```python
from build123d import *

# Parameters (mm, degrees)
SKETCH1_W           = 55
SKETCH1_H           = 55
SKETCH1_W_2         = 12
SKETCH1_H_2         = 13.5
BOSS_EXTRUDE1_DEPTH = 8
SKETCH2_W           = 55
SKETCH2_H           = 55
BOSS_EXTRUDE7_DEPTH = 12
SKETCH2_5_W         = 23.6
SKETCH2_5_H         = 7
SKETCH2_5_W_2       = 47
BOSS_EXTRUDE8_DEPTH = 8
SKETCH6_R           = 3.15
CUT_EXTRUDE1_DEPTH  = 44.732139211
SKETCH7_W           = 24.995653022
SKETCH7_H           = 4
CUT_EXTRUDE3_DEPTH  = 4


with BuildPart() as part:
    # Sketch1 → Boss-Extrude1 (new body)
    with BuildSketch(Plane(origin=(0, 0, 0), x_dir=(1, 0, 0), z_dir=(0, 1, 0))):
        Rectangle(SKETCH1_W, SKETCH1_H)
        with Locations((0, 16.75)):
            Rectangle(SKETCH1_W_2, SKETCH1_H_2, mode=Mode.SUBTRACT)
        with Locations((17.5, 0)):
            Rectangle(SKETCH1_W_2, SKETCH1_H_2, mode=Mode.SUBTRACT)
        with Locations((-17.5, 0)):
            Rectangle(SKETCH1_W_2, SKETCH1_H_2, mode=Mode.SUBTRACT)
        with Locations((0, -16.75)):
            Rectangle(SKETCH1_W_2, SKETCH1_H_2, mode=Mode.SUBTRACT)
    extrude(amount=BOSS_EXTRUDE1_DEPTH)

    # Sketch2 → Boss-Extrude7 (add)
    with BuildSketch(Plane.XZ):
        Rectangle(SKETCH2_W, SKETCH2_H)
        Polygon((-23.5, 23.5), (-6, 23.5), (6, 23.5), (23.5, 23.5), (23.5, 6.75), (23.5, 3.5), (23.5, -3.5), (23.5, -6.75), (23.5, -23.5), (6, -23.5), (-6, -23.5), (-23.5, -23.5), (-23.5, -6.75), (-23.5, -3.5), (-23.5, 3.5), (-23.5, 6.75), align=None, mode=Mode.SUBTRACT)
    extrude(amount=BOSS_EXTRUDE7_DEPTH)

    # Sketch2_5 → Boss-Extrude8 (add)
    with BuildSketch(Plane.XZ):
        with Locations((-0.1, 16.75)):
            Rectangle(SKETCH2_5_W, SKETCH2_5_H)
        Rectangle(SKETCH2_5_W_2, SKETCH2_5_H)
        with Locations((-0.1, -16.75)):
            Rectangle(SKETCH2_5_W, SKETCH2_5_H)
    extrude(amount=BOSS_EXTRUDE8_DEPTH)

    # Sketch6 → Cut-Extrude1 (cut, through all)
    with BuildSketch(Plane.XZ.offset(12)):
        with Locations(Location((-23.5, 23.5, 0), (0, 0, 270))):
            Circle(SKETCH6_R)
        with Locations(Location((23.5, 23.5, 0), (0, 0, 270))):
            Circle(SKETCH6_R)
        with Locations(Location((-23.5, -23.5, 0), (0, 0, 270))):
            Circle(SKETCH6_R)
        with Locations(Location((23.5, -23.5, 0), (0, 0, 270))):
            Circle(SKETCH6_R)
    extrude(amount=-CUT_EXTRUDE1_DEPTH, mode=Mode.SUBTRACT)

    # Sketch7 → Cut-Extrude3 (cut)
    with BuildSketch(Plane(origin=(27.5, 0, 0), x_dir=(0, 0, -1), z_dir=(1, 0, 0))):
        with Locations((0, -10)):
            Rectangle(SKETCH7_W, SKETCH7_H)
    extrude(amount=-CUT_EXTRUDE3_DEPTH, mode=Mode.SUBTRACT)


solid = part.part
```
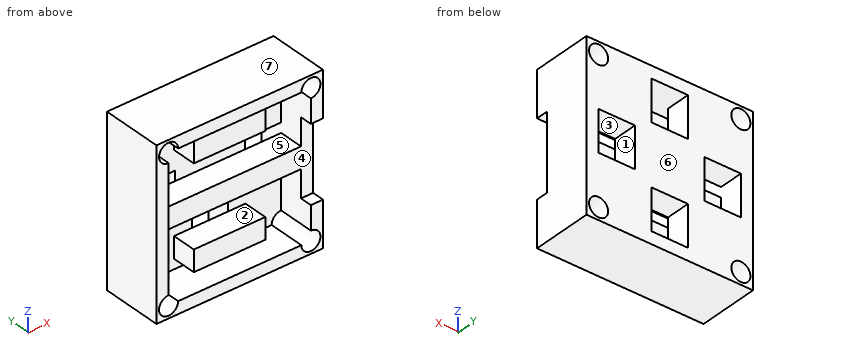
The listing builds one solid part. Answer for the finished solid, in the listing's coordinates (mm). Face numbers are marked on the shaded views. A direction names the side the tool comes from. Coordinates: 2 decimals unless noted, no trailing zeros. Order: outer loops, then holes, each group sorted by start corner. A loop starts at its lowest first (then second) coordinate and runs counter-clockwise, first axis right, second up. Notation, with made-up numbers: M 21.5,78.25 L 35.5,78.25 A33 ccw 35.5,117.25 Z; hole C 10.5,79 d8. An arc over 180 degrees is marked long. Answer as a JSON object with one key per item and string values. Group by question number.
1. Flat-ended cylindrical pins translate along their axes: P1, Ø5, axis at x = 18, z = 0, coming from the -Y side; P2, Ø5.5, axis at x = 0.5, z = -17, coming from the +Y side. Find the tip coordinate at first contact, or state that the pin passes through.
2. Determine the mould class of the marked faces 5, 6 and 7 for opening direction Z: released by +Z, released by -Z, zero draft, split by the parting line, or undercut.
3. A tool of negligible diameter and unlimited length cuts with its end or side. For the marked faces 1, 2, 3 and 4, from which of +Z, -Z, +X, -X, +Y, -Y can it reach the whole face along a straight path? Write none if from no direction.
4. Straight lines are drawn through the part: line 1 (Z direction, x = -8.5, y = -4.75); line 2 (X direction, y = 6.5, z = 3.5); line 3 (Z direction, x = 6, y = -10.25). For each, find the intervals that lie inside material, in ascending order.
5. Section A-A on x = 17 is taken. Write down the section's boundary in (y, z).
6. Section C-C on z = -6 is taken. Write down the section's boundary in (x, y).
7. Section D-D on x = -3.5 is taken. Write down the section's boundary in (y, z), then the cut area to 3 significant figures.
8. Section B-B on y = -2.25 is taken. Write down the section's boundary in (x, z).
Values follow:
{
 "1": {"P1": "y = -8", "P2": "y = 0"},
 "2": {"face 5": "undercut", "face 6": "zero draft", "face 7": "released by +Z"},
 "3": {"face 1": "+Y", "face 2": "-Y", "face 3": "+Y, -Y", "face 4": "+X, -Y"},
 "4": {"line 1": "-27.5 to -23.5, -20.25 to -13.25, -3.5 to 3.5, 13.25 to 20.25, 23.5 to 27.5", "line 2": "-27.5 to -23.5, -11.5 to 11.5, 23.5 to 27.5", "line 3": "-27.5 to -23.5, 23.5 to 27.5"},
 "5": {"outline": "M -12,-27.5 L 8,-27.5 L 8,-6.75 L 0,-6.75 L 0,-23.5 L -12,-23.5 Z; M -12,23.5 L 0,23.5 L 0,6.75 L 8,6.75 L 8,27.5 L -12,27.5 Z; M -8,-3.5 L 0,-3.5 L 0,3.5 L -8,3.5 Z"},
 "6": {"outline": "M -27.5,-12 L -23.5,-12 L -23.5,8 L -27.5,8 Z; M -11.5,0 L 11.5,0 L 11.5,8 L -11.5,8 Z; M 23.5,-8 L 27.5,-8 L 27.5,8 L 23.5,8 Z"},
 "7": {"outline": "M -12,-27.5 L 8,-27.5 L 8,-23.5 L -12,-23.5 Z; M -12,23.5 L 8,23.5 L 8,27.5 L -12,27.5 Z; M -8,-20.25 L 0,-20.25 L 0,-13.25 L -8,-13.25 Z; M -8,-3.5 L 0,-3.5 L 0,-10 L 8,-10 L 8,10 L 0,10 L 0,3.5 L -8,3.5 Z; M -8,13.25 L 0,13.25 L 0,20.25 L -8,20.25 Z", "area": "488 mm2"},
 "8": {"outline": "M -27.5,-27.5 L 27.5,-27.5 L 27.5,27.5 L -27.5,27.5 Z; M -11.9,-20.25 L 11.7,-20.25 L 11.7,-13.25 L -11.9,-13.25 Z; M -11.9,13.25 L 11.7,13.25 L 11.7,20.25 L -11.9,20.25 Z; hole M -23.5,-20.35 A3.15 ccw long -20.35,-23.5 L 20.35,-23.5 A3.15 ccw long 23.5,-20.35 L 23.5,-3.5 L -23.5,-3.5 Z; hole M -23.5,3.5 L 23.5,3.5 L 23.5,20.35 A3.15 ccw long 20.35,23.5 L -20.35,23.5 A3.15 ccw long -23.5,20.35 Z"}
}
